Work out the finished part from the listing and answer in its coordinate system (mm). A direction names the side the tool comes from. Round coordinates to 2 decimals unless told otherwise and drop trailing zeros. Write each loop counter-clockwise with the first axis right and the second up, starting at its lowest first coordinate (ties: lowest second). Pieces come first, ordered by that corner, then holes. Notation, with made-up numbers: (48.5, -23) -> (94.5, -23) arc R34 cw to (94.5, 15) -> close; hole circle Ø1 at (-30.75, 75.25). An arc over 180 degrees is marked (long way). One line per item, written item: value.
```python
from build123d import *

# Parameters (mm, degrees)
BOSS_EXTRUDE1_DEPTH      = 2
BOSS_EXTRUDE1_DEPTH_BACK = 9
SKETCH1_W                = 46.35
SKETCH1_H                = 60
SKETCH1_R                = 2
SKETCH2_W                = 30
SKETCH2_H                = 30
CUT_EXTRUDE1_DEPTH       = 6.35
SKETCH4_R                = 2
BOSS_EXTRUDE4_DEPTH      = 0.85
FILLET1_R                = 5


with BuildPart() as part:
    # Sketch1 → Boss-Extrude1 (new, two sides: drawn at the far end of the back side and taken through both)
    with BuildSketch(Plane.XY.offset(-BOSS_EXTRUDE1_DEPTH_BACK)):
        Rectangle(SKETCH1_W, SKETCH1_H)
        with Locations((-17.071067812, 17.071067812)):
            Circle(SKETCH1_R, mode=Mode.SUBTRACT)
        with Locations((-17.071067812, -17.071067812)):
            Circle(SKETCH1_R, mode=Mode.SUBTRACT)
        with Locations((17.071067812, -17.071067812)):
            Circle(SKETCH1_R, mode=Mode.SUBTRACT)
        with Locations((17.071067812, 17.071067812)):
            Circle(SKETCH1_R, mode=Mode.SUBTRACT)
        with Locations((0, 25.060622825)):
            Circle(SKETCH1_R, mode=Mode.SUBTRACT)
        with Locations((0, -25.060622825)):
            Circle(SKETCH1_R, mode=Mode.SUBTRACT)
    extrude(amount=BOSS_EXTRUDE1_DEPTH + BOSS_EXTRUDE1_DEPTH_BACK)

    # Sketch2 → Cut-Extrude1 (cut)
    with BuildSketch(Plane(origin=(0, 0, -9), x_dir=(-1, 0, 0), z_dir=(0, 0, -1))):
        Rectangle(SKETCH2_W, SKETCH2_H)
    extrude(amount=-CUT_EXTRUDE1_DEPTH, mode=Mode.SUBTRACT)

    # Sketch4 → Boss-Extrude4 (add)
    with BuildSketch(Plane(origin=(0, 0, -9), x_dir=(-1, 0, 0), z_dir=(0, 0, -1))):
        with Locations((-17.071067812, 17.071067812)):
            Circle(SKETCH4_R)
        with Locations((17.071067812, 17.071067812)):
            Circle(SKETCH4_R)
        with Locations((-17.071067812, -17.071067812)):
            Circle(SKETCH4_R)
        with Locations((17.071067812, -17.071067812)):
            Circle(SKETCH4_R)
    extrude(amount=-BOSS_EXTRUDE4_DEPTH)

    # Fillet1
    fillet1_edges = [part.edges().sort_by_distance(p)[0] for p in [
        (-23.175, -30, -3.5),
        (-23.175, 30, -3.5),
        (23.175, 30, -3.5),
        (23.175, -30, -3.5),
    ]]
    fillet(fillet1_edges, radius=FILLET1_R)


solid = part.part
```
(1) Flat-ended cylindrical pins translate along their axes: pin 1 Ø1.2 at (x, y) = (-17.5, -16.5) entering from +Z; pin 2 Ø15 at (x, y) = (-4, -6.5) entering from -Z; pin 3 Ø2.5 at (x, y) = (0, 25.06) entering from +Z (3 decimals). Find the tip coordinate at first contact, or state that the pin passes through.
Reported:
pin 1: stops at z = -8.15
pin 2: stops at z = -2.65
pin 3: passes through
(2) Find section C-C on z = -1.75. Give the vertices of the cut face in (x, y) (3 decimals), plus the area to 3 significant figures.
Reported:
outline: (-23.175, -25) arc R5 ccw to (-18.175, -30) -> (18.175, -30) arc R5 ccw to (23.175, -25) -> (23.175, 25) arc R5 ccw to (18.175, 30) -> (-18.175, 30) arc R5 ccw to (-23.175, 25) -> close; hole circle Ø4 at (-17.071, -17.071); hole circle Ø4 at (-17.071, 17.071); hole circle Ø4 at (0, -25.061); hole circle Ø4 at (0, 25.061); hole circle Ø4 at (17.071, -17.071); hole circle Ø4 at (17.071, 17.071)
area: 2,680 mm2
(3) For a pull along Y with two mould halves and no side action, classify faces 4 (the face through (0, 30, -4)), 5 (the face through (0, -30, -4)), 6 (the face through (-23.175, 0, -4)), 7 (the face through (-15.163, -16.47, -3.146)) as pulls with the +Y half, pulls with the -Y half, needs draft (parallel to the pull), parting line crosses it, or undercut.
Reported:
face 4: pulls with the +Y half
face 5: pulls with the -Y half
face 6: needs draft
face 7: undercut
(4) Find section D-D on y = -6. Give the vertices of the cut face in (x, z) (3 decimals).
Reported:
outline: (-23.175, -9) -> (-15, -9) -> (-15, -2.65) -> (15, -2.65) -> (15, -9) -> (23.175, -9) -> (23.175, 2) -> (-23.175, 2) -> close
(5) Find section B-B on x = 6. Give the vertices of the cut face in (y, z).
Reported:
outline: (-30, -9) -> (-15, -9) -> (-15, -2.65) -> (15, -2.65) -> (15, -9) -> (30, -9) -> (30, 2) -> (-30, 2) -> close
(6) A tool of negligible diameter and unlimited length cuts with its end or side. For faces 1 (the face through (-17, 17, -8.15)), 2 (the face through (0, 0, -2.65)), 3 (the face through (0, 0, 2)), from which of +Z, -Z, +X, -X, +Y, -Y can it reach the whole face along a straight path? Write none if from no direction.
Reported:
face 1: +Z
face 2: -Z
face 3: +Z, +X, -X, +Y, -Y
(7) Find section A-A on x = 0. Give the vertices of the cut face in (y, z).
Reported:
outline: (-30, -9) -> (-27.06, -9) -> (-27.06, 2) -> (-30, 2) -> close; (-23.06, -9) -> (-15, -9) -> (-15, -2.65) -> (15, -2.65) -> (15, -9) -> (23.06, -9) -> (23.06, 2) -> (-23.06, 2) -> close; (27.06, -9) -> (30, -9) -> (30, 2) -> (27.06, 2) -> close
(8) Consider probe 1 along Y at (x, z) = (0, -2.25); probe 2 along Y at (x, z) = (-13, -2.75); probe 3 along Y at (x, z) = (-17.5, -1.5). Determine where each line is inside the solid, lowest interval first.
Reported:
probe 1: y = -30 to -27.06, -23.06 to 23.06, 27.06 to 30
probe 2: y = -30 to -15, 15 to 30
probe 3: y = -30 to -19.02, -15.12 to 15.12, 19.02 to 30
